Part model, mm, in its own coordinate system. A direction names the side the tool comes from. Round coordinates to 2 decimals unless told otherwise and drop trailing zeros. Write each loop counter-clockwise with the first axis right and the second up, starting at its lowest first coordinate (ties: lowest second). Pieces come first, ordered by that corner, then holes. Notation, with made-up numbers: (33, -19.5) -> (54, -19.5) arc R17 ccw to (54, 0.5) -> close; hole circle Ø11 at (71.5, 35). An arc over 180 degrees is marked (long way). Use CSV: the item, a comma, the result in double quotes. Start each with the question number.
(1) Saw through at D-D (z = -324). Give the cut face in (x, y).
(2) Drop flat-ended pins along their axis: pin 1 (5 mm diameter, centred on x = -75.5, y = -60.5, fed in from -Z); pin 2 (10 mm diameter, centred on y = -22, z = -408.5, fed in from +X); pin 3 (3 mm diameter, centred on x = -16, z = -492, fed in from +Y); pin 4 (4 mm diameter, centred on x = 5.5, y = -70.5, fed in from +Z). Give the stop position or say it passes through.
(3) Two-plate mould, pull along X, no slides. Class faces 1 (the flat face through (-100, 3, -332)), 2 (the cylindrical face through (31.099, 3.042, -179.988)), 3 (the flat face through (1, -36, -395)): released by +X, released by -X, zero draft, split by the parting line, or undercut.
(4) Which spindle directions (+Z, -Z, +X, -X, +Y, -Y) get a long thin tool onto all of the face, cutting with end or side? Do faces 4 (the flat face through (1, -37, -401)), 5 (the flat face through (1, 0, -235)), 6 (the flat face through (100, -45.9, -400.7)). Say none if no direction does.
(5) Saw through at B-B (x = 30). Give the cut face in (y, z).
(6) Probe line 1 (Z direction, x = 24, y = -54.5); line 2 (Y direction, x = -75, z = -599); line 3 (Y direction, x = 57.5, z = -518). List the from-to ranges inside material, lowest first. Write a range as [from, to].
(7) Saw through at A-A (z = -112). Give the cut face in (x, y), plus the area to 3 significant figures.
(8) Saw through at C-C (y = -37). Give the cut face in (x, z).
```python
from build123d import *

# Parameters (mm, degrees)
SM_BASE_FLANGE_1_DEPTH = 100
CUT_EXTRUDE_1_REACH    = 696.392


# Sheet-metal steps are written as plain solids
with BuildPart() as part:
    # Sketch 1 → 基体-法兰1 (new, symmetric)
    with BuildSketch(Plane(origin=(0, 0, 0), x_dir=(0, 0, -1), z_dir=(1, 0, 0))):
        with BuildLine():
            Line((0, 0), (389, 0))
            ThreePointArc((389, 0), (393.242640687, -1.757359313), (395, -6))
            Line((395, -6), (395, -66.197173462))
            ThreePointArc((395, -66.197173462), (397.324227007, -73.295019402), (403.396569497, -77.643364471))
            Line((403.396569497, -77.643364471), (665, -160))
            Line((665, -160), (666.801715251, -154.276904496))
            Line((666.801715251, -154.276904496), (405.198284749, -71.920268967))
            ThreePointArc((405.198284749, -71.920268967), (402.162113503, -69.746096432), (401, -66.197173462))
            Line((401, -66.197173462), (401, -6))
            ThreePointArc((401, -6), (397.485281374, 2.485281374), (389, 6))
            Line((389, 6), (0, 6))
            Line((0, 6), (0, 0))
        make_face()
    extrude(amount=SM_BASE_FLANGE_1_DEPTH, both=True)

    # 草图4 → 切除-拉伸1 (cut, up to next)
    with BuildSketch(Plane(origin=(0, 6, 0), x_dir=(1, 0, 0), z_dir=(0, 1, 0)), mode=Mode.PRIVATE) as cut_extrude_1_sk1:
        with BuildLine():
            Line((-20, 130), (-20, 46.188021535))
            Line((-20, 46.188021535), (-100, 0))
            Line((-100, 0), (100, 0))
            Line((100, 0), (100, 95))
            Line((100, 95), (80, 95))
            Line((80, 95), (80, 130))
            ThreePointArc((80, 130), (30, 180), (-20, 130))
        make_face()
    cut_extrude_1_tool1 = extrude(cut_extrude_1_sk1.sketch, amount=-CUT_EXTRUDE_1_REACH, mode=Mode.PRIVATE) & part.part
    add(cut_extrude_1_tool1.solids().sort_by_distance((28.66293, 6, -75.336076))[0], mode=Mode.SUBTRACT)


solid = part.part
```
Answers:
1,outline,"(-100, 0) -> (100, 0) -> (100, 6) -> (-100, 6) -> close"
2,pin 1,"stops at z = -401"
2,pin 2,"passes through"
2,pin 3,"stops at y = -98.77"
2,pin 4,"stops at z = -395.22"
3,face 1,"released by -X"
3,face 2,"undercut"
3,face 3,"zero draft"
4,face 4,"-Z, +X, -X, +Y"
4,face 5,"+Z, +X, -X, -Y"
4,face 6,"+Z, -Z, +X, +Y, -Y"
5,outline,"(-160, -665) -> (-154.28, -666.8) -> (-71.92, -405.2) arc R6 cw to (-66.2, -401) -> (-6, -401) arc R12 ccw to (6, -389) -> (6, -180) -> (0, -180) -> (0, -389) arc R6 cw to (-6, -395) -> (-66.2, -395) arc R12 ccw to (-77.64, -403.4) -> close"
6,line 1,"z = [-401, -395]"
6,line 2,"y = [-139.22, -132.93]"
6,line 3,"y = [-113.72, -107.43]"
7,outline,"(-100, 0) -> (-20, 0) -> (-20, 6) -> (-100, 6) -> close; (80, 0) -> (100, 0) -> (100, 6) -> (80, 6) -> close"
7,area,"600 mm²"
8,outline,"(-100, -401) -> (100, -401) -> (100, -395) -> (-100, -395) -> close"
